```python
from build123d import *

# Parameters (mm, degrees)
SKETCH1_R               = 6.985
BOSS_EXTRUDE1_DEPTH     = 6.35
SKETCH3_R               = 4.7625
CUT_EXTRUDE1_DEPTH      = 63.5
SKETCH5_W               = 76.2
SKETCH5_H               = 13.97
BOSS_EXTRUDE2_DEPTH     = 101.6
SKETCH6_W               = 50.8
SKETCH6_H               = 95.25
CUT_EXTRUDE2_DEPTH      = 116.325510621
SKETCH7_R               = 4.7625
CUT_EXTRUDE3_DEPTH      = 115.689156964
CUT_EXTRUDE4_DEPTH      = 126.436209784
CUT_EXTRUDE4_DEPTH_BACK = 19.05
SKETCH8_R               = 4.7625


with BuildPart() as part:
    # Sketch1 → Boss-Extrude1 (new body)
    with BuildSketch(Plane(origin=(0, 0, 0), x_dir=(1, 0, 0), z_dir=(0, 1, 0))):
        with Locations(Location((0, 0, 0), (0, 0, 270))):
            Circle(SKETCH1_R)
    extrude(amount=-BOSS_EXTRUDE1_DEPTH)

    # Sketch3 → Cut-Extrude1 (cut)
    with BuildSketch(Plane(origin=(0, 0, 0), x_dir=(1, 0, 0), z_dir=(0, 1, 0))):
        with Locations(Location((0, 0, 0), (0, 0, 270))):
            Circle(SKETCH3_R)
    extrude(amount=-CUT_EXTRUDE1_DEPTH, mode=Mode.SUBTRACT)

    # Sketch5 → Boss-Extrude2 (add)
    with BuildSketch(Plane(origin=(0, -6.35, 0), x_dir=(-1, 0, 0), z_dir=(0, -1, 0))):
        Rectangle(SKETCH5_W, SKETCH5_H)
    extrude(amount=BOSS_EXTRUDE2_DEPTH)

    # Sketch6 → Cut-Extrude2 (cut, through all)
    with BuildSketch(Plane(origin=(0, 0, -6.985), x_dir=(-1, 0, 0), z_dir=(0, 0, -1))):
        with Locations((0, -60.325)):
            Rectangle(SKETCH6_W, SKETCH6_H)
    extrude(amount=-CUT_EXTRUDE2_DEPTH, mode=Mode.SUBTRACT)

    # Sketch7 → Cut-Extrude3 (cut, through all)
    with BuildSketch(Plane(origin=(0, 0, 0), x_dir=(1, 0, 0), z_dir=(0, 1, 0))):
        with Locations(Location((0, 0, 0), (0, 0, 270))):
            Circle(SKETCH7_R)
    extrude(amount=-CUT_EXTRUDE3_DEPTH, mode=Mode.SUBTRACT)

    # Sketch8 → Cut-Extrude4 (cut, two sides: drawn at the far end of the back side and taken through both)
    with BuildSketch(Plane.ZY.offset(-25.4).offset(-CUT_EXTRUDE4_DEPTH_BACK)):
        with Locations((0, -79.375)):
            Circle(SKETCH8_R)
    extrude(amount=CUT_EXTRUDE4_DEPTH + CUT_EXTRUDE4_DEPTH_BACK, mode=Mode.SUBTRACT)


solid = part.part
```
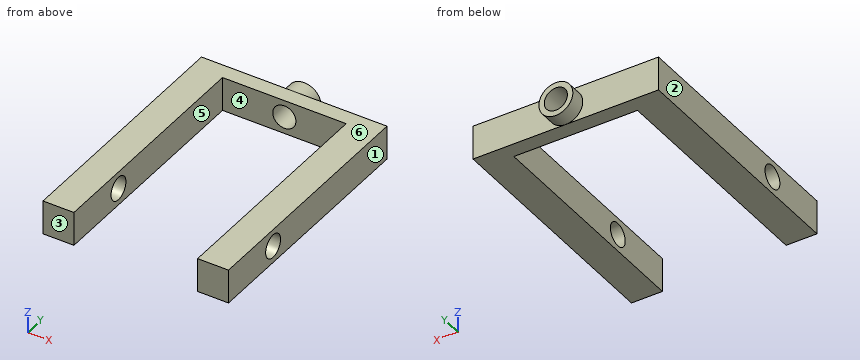
Here's how the part is built. I have some questions about the finished solid (model axes, mm). Face numbers are marked on the shaded views. A direction names the side the tool comes from. Coordinates: 2 decimals unless noted, no trailing zeros. Order: outer loops, then holes, each group sorted by start corner. A loop starts at its lowest first (then second) coordinate and runs counter-clockwise, first axis right, second up.
Item 1: I need wall thicknesses on probe 1 along X at (y, z) = (-4, 0) (1 decimal); probe 2 along X at (y, z) = (-53, 2.25); probe 3 along Y at (x, z) = (-31.25, 0). Which ranges of each line are inside material? Lowest first, please.
Response values:
probe 1: x = -7 to -4.8, 4.8 to 7
probe 2: x = -38.1 to -25.4, 25.4 to 38.1
probe 3: y = -107.95 to -84.14, -74.61 to -6.35
Item 2: Thinking about a two-plate mould opening in X: for the marked faces 1, 2, 3 and 4, which applies, pulls with the +X half, pulls with the -X half, needs draft (parallel to the pull), parting line crosses it, or undercut?
Response values:
face 1: pulls with the +X half
face 2: pulls with the -X half
face 3: needs draft
face 4: undercut
Item 3: If we section it at A-A, the plane y = -69.5: List the corners of the cut face in (x, z) for me (3 decimals).
Response values:
outline: (-38.1, -6.985) - (-25.4, -6.985) - (-25.4, 6.985) - (-38.1, 6.985) - close; (25.4, -6.985) - (38.1, -6.985) - (38.1, 6.985) - (25.4, 6.985) - close
Item 4: Which directions (+Z, -Z, +X, -X, +Y, -Y) give clear straight access to the entire face, cutting with the end or side of a thin tool? Please do the marked faces 5 and 6.
Response values:
face 5: +Z, -Z, -Y
face 6: +Z, +X, -X, +Y, -Y
Item 5: If we section it at B-B, the plane z = 0: Give the number of separate pieces and of enclosed holes in the cut face, then the cut area to 3 significant figures.
Response values:
separate pieces: 4
enclosed holes: 0
area: 2,630 mm2
Item 6: I'm going to push flat-ended pins straight in: pin 1 Ø4 at (x, z) = (7, -5.5) entering from -Y; pin 2 Ø2 at (x, z) = (20.5, -4) entering from +Y. Where does each tip first touch, or does it pass through?
Response values:
pin 1: stops at y = -12.7
pin 2: stops at y = -6.35
